Read the model definition and answer for the solid it produces. Units are mm, in the model's axes. Face numbers are marked on the shaded views. A direction names the side the tool comes from. Coordinates: 2 decimals unless noted, no trailing zeros. Loops run counter-clockwise (first coordinate to the right, second up) from the corner with the lowest first, then second, coordinate; pieces in that order, holes last. Notation, with made-up numbers: (0.5, -25.5) - (8.5, -25.5) arc R26 cw to (8.5, 12.5) - close; hole circle Ø1 at (29.5, -39). An arc over 180 degrees is marked (long way). One line per question, with ' | ' between items. Start each with the question number.
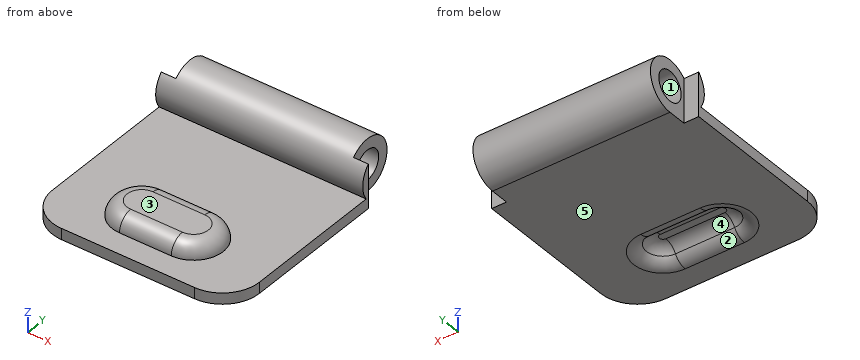
```python
from build123d import *

# Parameters (mm, degrees)
BOSS_EXTRUDE1_DEPTH      = 14
BOSS_EXTRUDE1_DEPTH_BACK = 14
SKETCH1_R                = 2
FILLET1_R                = 5
BOSS_EXTRUDE2_DEPTH      = 2
FILLET2_R                = 2
CUT_EXTRUDE1_DEPTH       = 2
FILLET3_R                = 2
FILLET4_R                = 2
SKETCH4_W                = 2
SKETCH4_H                = 6
CUT_EXTRUDE2_DEPTH       = 32.208973069


# Some blends are built 0.0001 mm under size
with BuildPart() as part:
    # Sketch1 → Boss-Extrude1 (new, two sides: drawn at the far end of the back side and taken through both)
    with BuildSketch(Plane(origin=(0, 0, 0), x_dir=(0, 0, -1), z_dir=(1, 0, 0)).offset(-BOSS_EXTRUDE1_DEPTH_BACK)):
        with BuildLine():
            Line((3.5, 0), (3.5, -27))
            Line((3.5, -27), (2, -27))
            Line((2, -27), (2, -2.872281323))
            ThreePointArc((2, -2.872281323), (-3.102418411, 1.620185175), (3.5, 0))
        make_face()
        Circle(SKETCH1_R, mode=Mode.SUBTRACT)
    extrude(amount=BOSS_EXTRUDE1_DEPTH + BOSS_EXTRUDE1_DEPTH_BACK)

    # Fillet1
    fillet1_edges = [part.edges().sort_by_distance(p)[0] for p in [
        (-14, -27, -2.75),
        (14, -27, -2.75),
    ]]
    fillet(fillet1_edges, radius=FILLET1_R)

    # Sketch2 → Boss-Extrude2 (add)
    with BuildSketch(Plane.XY.offset(-2)):
        with BuildLine():
            Line((-3.5, -15.881230087), (3.5, -15.881230087))
            ThreePointArc((3.5, -15.881230087), (7.5, -19.881230087), (3.5, -23.881230087))
            Line((3.5, -23.881230087), (-3.5, -23.881230087))
            ThreePointArc((-3.5, -23.881230087), (-7.5, -19.881230087), (-3.5, -15.881230087))
        make_face()
    extrude(amount=BOSS_EXTRUDE2_DEPTH)

    # Fillet2
    fillet2_edges = [part.edges().sort_by_distance(p)[0] for p in [
        (-7.5, -19.881230087, 0),
        (0, -15.881230087, 0),
        (7.5, -19.881230087, 0),
        (0, -23.881230087, 0),
    ]]
    fillet(fillet2_edges, radius=FILLET2_R - 0.0001)  # a hair under: the kernel refuses the full size

    # Sketch3 → Cut-Extrude1 (cut)
    with BuildSketch(Plane(origin=(0, 0, -3.5), x_dir=(-1, 0, 0), z_dir=(0, 0, -1))):
        with BuildLine():
            Line((-4, -17.437696963), (4, -17.437696963))
            ThreePointArc((4, -17.437696963), (6.5, -19.937696963), (4, -22.437696963))
            Line((4, -22.437696963), (-4, -22.437696963))
            ThreePointArc((-4, -22.437696963), (-6.5, -19.937696963), (-4, -17.437696963))
        make_face()
    extrude(amount=-CUT_EXTRUDE1_DEPTH, mode=Mode.SUBTRACT)

    # Fillet3
    fillet3_edges = [part.edges().sort_by_distance(p)[0] for p in [
        (-6.5, -19.937696963, -1.5),
        (0, -22.437696963, -1.5),
        (6.5, -19.937696963, -1.5),
        (0, -17.437696963, -1.5),
    ]]
    fillet(fillet3_edges, radius=FILLET3_R - 0.0001)  # a hair under: the kernel refuses the full size

    # Fillet4
    # the kernel refuses this fillet: 2 mm, written as the material it takes off along each edge
    with BuildSketch(Plane(origin=(4, -19.937696963, -3.5), x_dir=(0, -1, 0), z_dir=(-1, 0, 0))) as fillet4_piece_1:
        with BuildLine():
            CenterArc((3.96414388, 2), FILLET4_R, 209.999172989, 60.000827011)
            Line((3.96414388, 0), (3.96414388, -0.2))
            Line((3.96414388, -0.2), (2.5, -0.2))
            Line((2.5, -0.2), (2.3, 0))
            ThreePointArc((2.3, 0), (2.3, 0.0001), (2.058872114, 0.900027501))
            Line((2.058872114, 0.900027501), (2.232078638, 1.000025001))
        make_face()
    revolve(axis=Axis((4, -19.937696963, -3.5), (0, 0, 1)), revolution_arc=180, mode=Mode.SUBTRACT)
    with BuildSketch(Plane(origin=(-4, -22.437696963, -3.5), x_dir=(0, 0.2587879267537998, 0.9659341638882383), z_dir=(1, 0, 0))) as fillet4_piece_2:
        with BuildLine():
            CenterArc((1.552965569, 1.931842448), FILLET4_R, 194.998154162, 60.000827011)
            Line((-0.378902759, 1.414266594), (-0.572089592, 1.362509009))
            Line((-0.572089592, 1.362509009), (-0.193186833, -0.051757585))
            Line((-0.193186833, -0.051757585), (0.051757585, -0.193186833))
            ThreePointArc((0.051757585, -0.193186833), (0.051854179, -0.193160954), (0.983525882, -0.193184245))
            Line((0.983525882, -0.193184245), (1.035293127, 0))
        make_face()
    extrude(amount=8, mode=Mode.SUBTRACT)
    with BuildSketch(Plane(origin=(-4, -19.937696963, -3.5), x_dir=(0, 1, 0), z_dir=(1, 0, 0))) as fillet4_piece_3:
        with BuildLine():
            CenterArc((3.96414388, 2), FILLET4_R, 209.999172989, 60.000827011)
            Line((2.232078638, 1.000025001), (2.058872114, 0.900027501))
            ThreePointArc((2.058872114, 0.900027501), (2.3, 0.0001), (2.3, 0))
            Line((2.3, 0), (2.5, -0.2))
            Line((2.5, -0.2), (3.96414388, -0.2))
            Line((3.96414388, -0.2), (3.96414388, 0))
        make_face()
    revolve(axis=Axis((-4, -19.937696963, -3.5), (0, 0, 1)), revolution_arc=180, mode=Mode.SUBTRACT)
    with BuildSketch(Plane(origin=(4, -17.437696963, -3.5), x_dir=(0, 1, 0), z_dir=(-1, 0, 0))) as fillet4_piece_4:
        with BuildLine():
            CenterArc((1.46414388, -2), FILLET4_R, 90, 60.000827011)
            Line((-0.267921362, -1.000025001), (-0.441127886, -0.900027501))
            ThreePointArc((-0.441127886, -0.900027501), (-0.2, -0.0001), (-0.2, 0))
            Line((-0.2, 0), (0, 0.2))
            Line((0, 0.2), (1.46414388, 0.2))
            Line((1.46414388, 0.2), (1.46414388, 0))
        make_face()
    extrude(amount=8, mode=Mode.SUBTRACT)

    # Sketch4 → Cut-Extrude2 (cut, through all)
    with BuildSketch(Plane(origin=(0, 0, -3.5), x_dir=(-1, 0, 0), z_dir=(0, 0, -1))):
        with Locations((-13, 0.5)):
            Rectangle(SKETCH4_W, SKETCH4_H)
        with Locations((13, 0.5)):
            Rectangle(SKETCH4_W, SKETCH4_H)
    extrude(amount=-CUT_EXTRUDE2_DEPTH, mode=Mode.SUBTRACT)


solid = part.part
```
1) The mould has two halves that part along X. Classify the marked faces 1 and 2: released by +X, released by -X, zero draft, split by the parting line, or undercut.
2) Given pin 1 Ø2 at (x, z) = (-13.5, 0.5) entering from +Y; pin 2 Ø2 at (y, z) = (-18, 2) entering from -X; pin 3 Ø3 at (y, z) = (-21.5, 1) entering from +X; pin 4 Ø12 at (x, y) = (2, -15) entering from +Z, each flat-ended and moving along its own axis, determine where each tip first touches the part or whether it passes through.
3) The part is cut by section D-D on y = -9.5. Write down the section's boundary in (x, z).
4) The part is cut by section C-C on z = 0.5. Write down the section's boundary in (x, y).
5) The part is cut by section B-B on z = -3. Write down the section's boundary in (x, y).
6) Which of the six approach directions +Z, -Z, +X, -X, +Y, -Y give full straight-line access (tool end or side, diameter ignored) to the marked faces 3, 4 and 5?
7) The part is cut by section A-A on y = 1.5. Write down the section's boundary in (x, z), and give its area (3 significant figures).
8) Find the intervals of material crossed by line 1 along Y through (x, z) = (11.75, 0); line 2 along Z through (x, y) = (-4.25, -24); line 3 along Y through (x, z) = (-0.25, -0.5), in increasing order. Write a range as from..to.
Answer below:
1) face 1: zero draft | face 2: undercut
2) pin 1: y = -2.5 | pin 2: through | pin 3: x = 6.52 | pin 4: z = 0
3) outline: (-14, -3.5) - (14, -3.5) - (14, -2) - (-14, -2) - close
4) outline: (-14, -3.46) - (14, -3.46) - (14, -2.5) - (12, -2.5) - (12, -1.94) - (-12, -1.94) - (-12, -2.5) - (-14, -2.5) - close; (-12, 1.94) - (12, 1.94) - (12, 3.46) - (-12, 3.46) - close
5) outline: (-14, -22) arc R5 ccw to (-9, -27) - (9, -27) arc R5 ccw to (14, -22) - (14, -2.5) - (12, -2.5) - (12, 1.8) - (-12, 1.8) - (-12, -2.5) - (-14, -2.5) - close; hole (-4, -22.58) - (4, -22.58) arc R2.64 ccw to (4, -17.3) - (-4, -17.3) arc R2.64 ccw to start
6) face 3: +Z, +X, -X, -Y | face 4: -Z | face 5: -Z, +X, -X, +Y, -Y
7) outline: (-12, -3.16) - (12, -3.16) - (12, -1.32) - (-12, -1.32) - close; (-12, 1.32) - (12, 1.32) - (12, 3.16) - (-12, 3.16) - close | area: 88.3 mm2
8) line 1: -3.5..-2, 2..3.5 | line 2: -3.5..-2 | line 3: -23.2..-16.56, -3.46..-1.94, 1.94..3.46
